Here's how the part is built. I have some questions about the finished solid (model axes, mm). A direction names the side the tool comes from. Give positions to 0.01 mm unless a question says otherwise; leave off trailing zeros. Loops run counter-clockwise (first coordinate to the right, second up) from the corner with the lowest first, then second, coordinate; pieces in that order, holes last.
Q1. Suppose I cut it at C-C (z = 27.5). List the corners of the cut face in (x, y) for me.
Q2. Thinking about a two-plate mould opening in Z: for faces 6 (the face through (6.4, 2, 39)), 7 (the face through (138.074, 25.311, 73.791)), 8 (the face through (71, 19, 95.72)), which applies, pulls with the +Z half, pulls with the -Z half, needs draft (parallel to the pull), parting line crosses it, or undercut?
Q3. Suppose I cut it at D-D (y = 35). List the corners of the cut face in (x, z) for me, and give its area (3 significant figures).
Q4. Suppose I cut it at B-B (x = 34.5). List the corners of the cut face in (y, z) for me.
Q5. I need wall thicknesses on probe 1 along Z at (x, y) = (66.5, 24); probe 2 along X at (y, z) = (3.5, 42.5); probe 3 along Z at (x, y) = (70, 9). Which ranges of each line are inside material? Lowest first, please.
Q6. I'm going to push flat-ended pins straight in: P1, Ø3, axis at x = 43.5, z = 75.5, coming from the +Y side; P2, Ø0.8, axis at x = 5.5, z = 49, coming from the -Y side; P3, Ø1, axis at y = 30.5, z = 77, coming from the +X side. Where does each tip first touch, or does it pass through?
Q7. For faces 1 (the face through (77.485, 16.319, 112.93)), 2 (the face through (138.074, 6.93, 73.79)), 3 (the face through (3.944, 25.311, 73.806)), 4 (the face through (75.015, 18.824, 103.295)), 5 (the face through (3, 25, 37)), which set-ups out of +Z, -Z, +X, -X, +Y, -Y let a thin tool reach every point of the face, with its end or its side?
```python
from build123d import *
from build123d.topology import SkipClean

# Parameters (mm, degrees)
EXTRUDE_1_DEPTH      = 2
EXTRUDE_2_DEPTH      = 10
CUT_EXTRUDE_1_DEPTH  = 5
SKETCH_4_W           = 126
SKETCH_4_H           = 3
EXTRUDE_4_DEPTH      = 37
EXTRUDE_5_DEPTH      = 27
SKETCH_6_R           = 4
EXTRUDE_6_DEPTH      = 110
SKETCH_7_W           = 8
SKETCH_7_H           = 92.720195249
CUT_EXTRUDE_2_DEPTH  = 25
EXTRUDE_7_DEPTH      = 5
EXTRUDE_7_DEPTH_BACK = 5
SKETCH_8_R           = 7


with BuildPart() as part:
    # Sketch 1 → Extrude 1 (new body)
    with BuildSketch(Plane(origin=(0, 0, 0), x_dir=(1, 0, 0), z_dir=(0, 1, 0))):
        with BuildLine():
            Line((0, 0), (0, -70.42))
            ThreePointArc((0, -70.42), (71, -98.800967575), (142, -70.42))
            Line((142, -70.42), (142, 0))
            Line((142, 0), (0, 0))
        make_face()
    extrude(amount=EXTRUDE_1_DEPTH)

    # Sketch 2 → Extrude 2 (add)
    with BuildSketch(Plane(origin=(0, 2, 0), x_dir=(1, 0, 0), z_dir=(0, 1, 0))):
        with BuildLine():
            Line((8, 0), (8, -77.287162725))
            ThreePointArc((8, -77.287162725), (3.912076489, -73.956009121), (0, -70.42))
            Line((0, -70.42), (0, 0))
            Line((0, 0), (8, 0))
        make_face()
        Polygon((134, -77.287162725), (134, 0), (142, 0), (142, -70.42), align=None)
    extrude(amount=EXTRUDE_2_DEPTH)

    # Sketch 3 → Cut-Extrude 1 (cut)
    with BuildSketch(Plane.XZ):
        Polygon((3.6, 0), (3.6, 73.687038217), (3.6, 76.02465485), (6.4, 76.02465485), (6.4, 0), align=None)
        Polygon((138.4, 0), (138.4, 73.687038217), (138.4, 76.02465485), (135.6, 76.02465485), (135.6, 0), align=None)
    extrude(amount=-CUT_EXTRUDE_1_DEPTH, mode=Mode.SUBTRACT)

    # Sketch 4 → Extrude 4 (add)
    with SkipClean():  # the faces are left unmerged after this step: merging them gives an invalid solid
        with BuildSketch(Plane(origin=(0, 2, 0), x_dir=(1, 0, 0), z_dir=(0, 1, 0))):
            with Locations((71, -1.5)):
                Rectangle(SKETCH_4_W, SKETCH_4_H)
            with BuildLine():
                Line((8, -73.460480837), (8, -77.287162725))
                ThreePointArc((8, -77.287162725), (71.023325312, -98.800964934), (134.036900158, -77.258620491))
                Line((134.036900158, -77.258620491), (134, -73.460480837))
                ThreePointArc((134, -73.460480837), (71, -95.800967575), (8, -73.460480837))
            make_face()
        extrude(amount=EXTRUDE_4_DEPTH)

    # Sketch 5 → Extrude 5 (add)
    with SkipClean():  # the faces are left unmerged after this step: merging them gives an invalid solid
        with BuildSketch(Plane(origin=(0, 12, 0), x_dir=(1, 0, 0), z_dir=(0, 1, 0))):
            Polygon((134, 0), (142, 0), (142, -70.42), (134.036900158, -77.258620491), (134, -73.460480837), (139, -69.16653713), (139, -3), (134, -3), align=None)
            Polygon((8, -3), (8, 0), (0, 0), (0, -70.42), (8, -77.287162725), (8, -73.460480837), (3, -69.168504133), (3, -3), align=None)
        extrude(amount=EXTRUDE_5_DEPTH)

    # Sketch 6 → Extrude 6 (add)
    with BuildSketch(Plane.XY.offset(3)):
        with Locations(Location((71.018450079, 19, 0), (0, 0, 180))):
            Circle(SKETCH_6_R)
    extrude(amount=EXTRUDE_6_DEPTH)

    # Sketch 7 → Cut-Extrude 2 (cut)
    with SkipClean():  # the faces are left unmerged after this step: merging them gives an invalid solid
        with BuildSketch(Plane(origin=(0, 39, 0), x_dir=(1, 0, 0), z_dir=(0, 1, 0))):
            with Locations((71.018450079, -49.360097624)):
                Rectangle(SKETCH_7_W, SKETCH_7_H)
        extrude(amount=-CUT_EXTRUDE_2_DEPTH, mode=Mode.SUBTRACT)

    # Sketch 8 → Extrude 7 (add, two sides: drawn at the far end of the back side and taken through both)
    with SkipClean():  # the faces are left unmerged after this step: merging them gives an invalid solid
        with BuildSketch(Plane.XY.offset(113).offset(-EXTRUDE_7_DEPTH_BACK)):
            with Locations((71.018450079, 19)):
                Circle(SKETCH_8_R)
        extrude(amount=EXTRUDE_7_DEPTH + EXTRUDE_7_DEPTH_BACK)


solid = part.part
```
Solutions:
1. outline: (0, 0) - (3.6, 0) - (3.6, 5) - (6.4, 5) - (6.4, 0) - (135.6, 0) - (135.6, 5) - (138.4, 5) - (138.4, 0) - (142, 0) - (142, 39) - (139, 39) - (139, 12) - (134, 12) - (134, 2) - (8, 2) - (8, 12) - (3, 12) - (3, 39) - (0, 39) - close
2. face 6: needs draft
2. face 7: pulls with the +Z half
2. face 8: undercut
3. outline: (0, 0) - (142, 0) - (142, 70.42) - (134.04, 77.26) arc R103 ccw to (8, 77.29) - (0, 70.42) - close; hole (3, 3) - (139, 3) - (139, 69.17) - (134, 73.46) arc R100 ccw to (8, 73.46) - (3, 69.17) - close
3. area: 1,280 mm2
4. outline: (0, 0) - (39, 0) - (39, 3) - (2, 3) - (2, 88.9) - (39, 88.9) - (39, 92.12) - (0, 92.12) - close
5. probe 1: z = 0 to 3, 95.7 to 98.7, 108 to 118
5. probe 2: x = 0 to 3.6, 6.4 to 8, 134 to 135.6, 138.4 to 142
5. probe 3: z = 0 to 3, 95.8 to 98.8
6. P1: stops at y = 2
6. P2: stops at y = 5
6. P3: stops at x = 134.92
7. face 1: +Z
7. face 2: +Z, +X, +Y
7. face 3: +Z, -X, +Y
7. face 4: none
7. face 5: +Y
